from build123d import *

# Parameters (mm, degrees)
F0_R     = 6
F0_R_2   = 5
F1_DEPTH = 8
F3_R     = 3.5
F3_R_2   = 1.5
F4_DEPTH = 5
F5_R     = 5
F6_DEPTH = 7
F7_R     = 1.5
F8_DEPTH = 25


with BuildPart() as f1:
    # F0 (on Front) → F1 (new body)
    with BuildSketch(Plane.XZ):
        Circle(F0_R)
        Circle(F0_R_2, mode=Mode.SUBTRACT)
        Circle(F0_R_2)
    extrude(amount=-F1_DEPTH)

    # F3 (on offset) → F4 (join)
    with BuildSketch(Plane.XZ.offset(-8)):
        Circle(F3_R)
        Circle(F3_R_2, mode=Mode.SUBTRACT)
        Circle(F3_R_2)
    extrude(amount=-F4_DEPTH)

    # F5 (on Front) → F6 (cut)
    with BuildSketch(Plane.XZ):
        Circle(F5_R)
    extrude(amount=-F6_DEPTH, mode=Mode.SUBTRACT)

    # F7 (on Front) → F8 (cut)
    with BuildSketch(Plane.XZ):
        Circle(F7_R)
    extrude(amount=-F8_DEPTH, mode=Mode.SUBTRACT)


solid = f1.part
Read the model definition and answer for the solid it produces. Units are mm, in the model's axes. A direction names the side the tool comes from. Give positions to 0.01 mm unless a question says otherwise; leave off trailing zeros. Loops run counter-clockwise (first coordinate to the right, second up) from the corner with the lowest first, then second, coordinate; pieces in that order, holes last. Notation, with made-up numbers: (31.5, 79.25) -> (63.5, 79.25) arc R7 ccw to (63.5, 85.25) -> close; hole circle Ø6 at (-11, 31.5). An arc over 180 degrees is marked (long way). Answer as CSV lines item,"result".
Item 1: Find section D-D on z = 2.75. Give the vertices of the cut face in (x, y).
Returned:
outline,"(-5.33, 0) -> (-4.18, 0) -> (-4.18, 7) -> (4.18, 7) -> (4.18, 0) -> (5.33, 0) -> (5.33, 8) -> (2.17, 8) -> (2.17, 13) -> (-2.17, 13) -> (-2.17, 8) -> (-5.33, 8) -> close"
Item 2: Consider line 1 (Z direction, x = 0, y = 10.1); line 2 (Z direction, x = 0, y = 2); line 3 (X direction, y = 6.5, z = 0.75). Determine where each line is inside the solid, lowest interval first. Write a range as [from, to].
Returned:
line 1,"z = [-3.5, -1.5], [1.5, 3.5]"
line 2,"z = [-6, -5], [5, 6]"
line 3,"x = [-5.95, -4.94], [4.94, 5.95]"
Item 3: Determine the mould class of faces 3 (the face through (3.233, 10.465, -1.341)), 4 (the face through (3, 8, -3)), 5 (the face through (-1.5, 9.96, 0.07)) for opening direction Z: +Z half, -Z half, draft (parallel to the pull), parting line (faces both ways), or undercut.
Returned:
face 3,"parting line"
face 4,"draft"
face 5,"undercut"
Item 4: For faces 1 (the face through (-4, 0, 4)), 2 (the face through (-1.2, 7, 1.2)), determine the directions among +Z, -Z, +X, -X, +Y, -Y from which every point of the face is accessible in a straight line to the end or side of a thin tool.
Returned:
face 1,"+Z, -Z, +X, -X, -Y"
face 2,"-Y"
Item 5: Find section C-C on y = 2.5. Give the vertices of the cut face in (x, z), plus the area to 3 significant figures.
Returned:
outline,"circle Ø12 at (0, 0); hole circle Ø10 at (0, 0)"
area,"34.6 mm²"
Item 6: Each of these flat-tipped pins is pushed along its axis until it touches: pin 1 (1.5 mm diameter, centred on x = -1, y = 7, fed in from -Z); pin 2 (1 mm diameter, centred on x = 2.5, y = 9, fed in from -Z). Where does it stop, or does it pass through?
Returned:
pin 1,"stops at z = -5.99"
pin 2,"stops at z = -2.87"
Item 7: Find section B-B on x = 0. Give the vertices of the cut face in (y, z), plus the area to 3 significant figures.
Returned:
outline,"(0, -6) -> (8, -6) -> (8, -3.5) -> (13, -3.5) -> (13, -1.5) -> (7, -1.5) -> (7, -5) -> (0, -5) -> close; (0, 5) -> (7, 5) -> (7, 1.5) -> (13, 1.5) -> (13, 3.5) -> (8, 3.5) -> (8, 6) -> (0, 6) -> close"
area,"43.0 mm²"
Item 8: Find section A-A on z = 0. Give the vertices of the cut face in (x, y), plus the area to 3 significant figures.
Returned:
outline,"(-6, 0) -> (-5, 0) -> (-5, 7) -> (-1.5, 7) -> (-1.5, 13) -> (-3.5, 13) -> (-3.5, 8) -> (-6, 8) -> close; (1.5, 7) -> (5, 7) -> (5, 0) -> (6, 0) -> (6, 8) -> (3.5, 8) -> (3.5, 13) -> (1.5, 13) -> close"
area,"43.0 mm²"
